For this review, use the dimensioned drawing (mm, ordinates from the lowest corner) and the shaded views. A direction names the side the tool comes from. Coordinates: 2 decimals unless noted, no trailing zeros. Loops run counter-clockwise (first coordinate to the right, second up) from the corner with the lowest first, then second, coordinate; pieces in that order, holes last. Notation, with made-up numbers: (-37.75, -24.75) - (-12.75, -24.75) arc R22 ccw to (-12.75, 1.25) - close; hole circle Ø1 at (3, 62). An arc over 180 degrees is marked (long way). Answer in a Markdown table with one row per item. Add a question column.
(1) We need section B-B, the plane y = 10. Write out the cut boundary in (x, z), plus the area to 3 significant figures.
(2) To check wall thickness, follow L1, parallel to X at y = 93, z = 25.5; L2, parallel to X at y = 81, z = 22; L3, parallel to Z at x = 18, y = 62.5. State the ranges of each line that lie inside material, in increasing order. Write a range as [from, to].
(3) The part is to be moulded in two halves that separate along Y. For the marked faces 1, 2, 3 and 4, say which applies: released by +Y, released by -Y, zero draft, split by the parting line, or undercut.
(4) We need section A-A, the plane z = 66. Write out the cut boundary in (x, y).
(5) We need section C-C, the plane x = 120. Write out the cut boundary in (y, z).
(6) Clearance check with flat-ended pins moving along their axes: pin 1 (2 mm diameter, centred on x = 39.5, y = 70, fed in from +Z); pin 2 (12.5 mm diameter, centred on y = 29.5, z = 17.5, fed in from +X); pin 3 (5.5 mm diameter, centred on x = 7.5, y = 52.5, fed in from +Z). State where each tip first meets the part, or that it passes through.
(7) We need section D-D, the plane z = 12. Write out the cut boundary in (x, y).
(8) For the marked faces 5, 6 and 7, list the 3-axis set-ups (+Z, -Z, +X, -X, +Y, -Y) from which the entire face can be reached by the end or side of a thin tool; tool diameter is ignored.
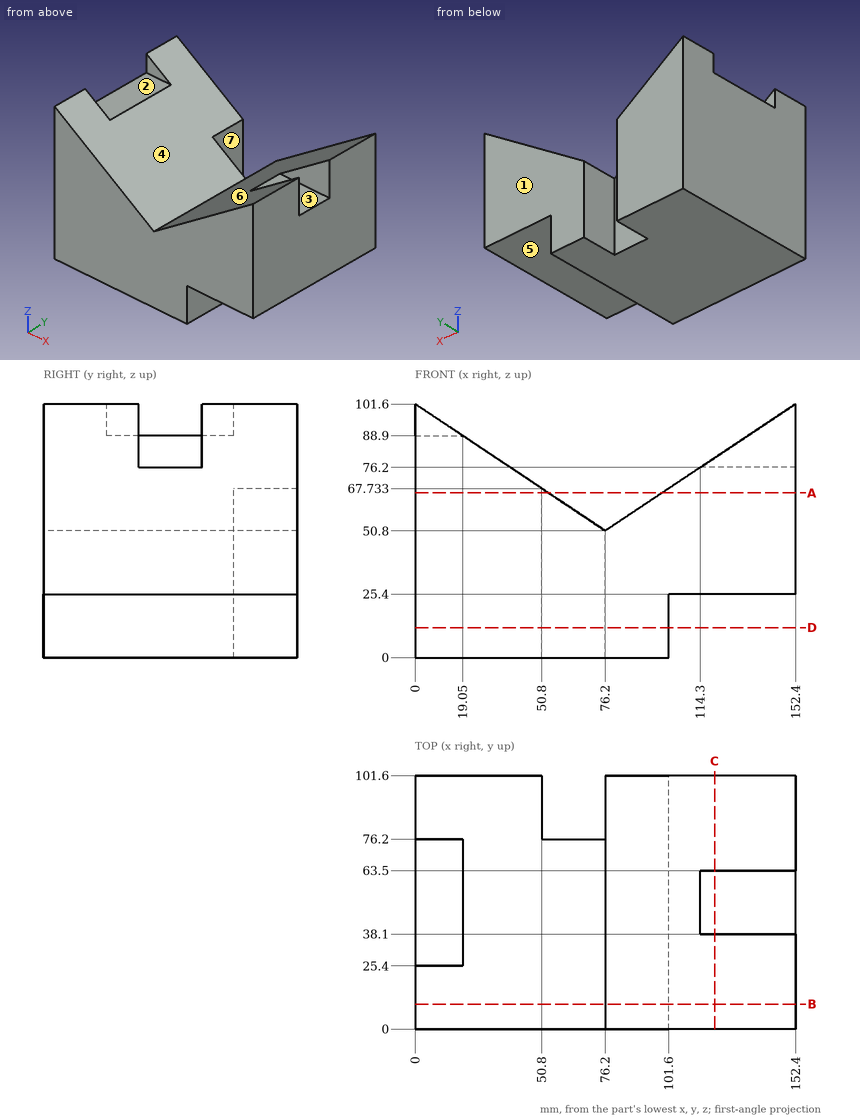
Responses:
| question | item | result |
|---|---|---|
| 1 | outline | (0, 0) - (101.6, 0) - (101.6, 25.4) - (152.4, 25.4) - (152.4, 101.6) - (76.2, 50.8) - (0, 101.6) - close |
| 1 | area | 10,300 mm2 |
| 2 | L1 | x = [0, 50.8], [76.2, 152.4] |
| 2 | L2 | x = [0, 50.8], [76.2, 101.6] |
| 2 | L3 | z = [0, 88.9] |
| 3 | face 1 | released by +Y |
| 3 | face 2 | undercut |
| 3 | face 3 | undercut |
| 3 | face 4 | zero draft |
| 4 | outline | (0, 0) - (53.4, 0) - (53.4, 76.2) - (50.8, 76.2) - (50.8, 101.6) - (0, 101.6) - close; (99, 0) - (152.4, 0) - (152.4, 101.6) - (99, 101.6) - close |
| 5 | outline | (0, 25.4) - (101.6, 25.4) - (101.6, 80) - (63.5, 80) - (63.5, 76.2) - (38.1, 76.2) - (38.1, 80) - (0, 80) - close |
| 6 | pin 1 | stops at z = 75.93 |
| 6 | pin 2 | stops at x = 101.6 |
| 6 | pin 3 | stops at z = 88.9 |
| 7 | outline | (0, 0) - (101.6, 0) - (101.6, 101.6) - (76.2, 101.6) - (76.2, 76.2) - (50.8, 76.2) - (50.8, 101.6) - (0, 101.6) - close |
| 8 | face 5 | -Z, +X, +Y, -Y |
| 8 | face 6 | +Z, +Y, -Y |
| 8 | face 7 | +Z, -Z, +Y |
